from build123d import *

# Parameters (mm, degrees)
SKETCH1_W           = 254
SKETCH1_H           = 38.1
BOSS_EXTRUDE1_DEPTH = 3.175
CUT_EXTRUDE1_DEPTH  = 10.414


with BuildPart() as part:
    # Sketch1 → Boss-Extrude1 (new body)
    with BuildSketch(Plane.XY):
        Rectangle(SKETCH1_W, SKETCH1_H)
    extrude(amount=BOSS_EXTRUDE1_DEPTH)

    # Sketch4 → Cut-Extrude1 (cut)
    with BuildSketch(Plane.XY.offset(3.175)):
        Polygon((-99.060120052, -9.6425385), (-99.060120052, 2.8223845), (-109.855060026, 9.054846), (-120.65, 2.8223845), (-120.65, -9.6425385), (-109.855060026, -15.875), align=None)
        Polygon((-76.200120052, -9.6425385), (-76.200120052, 2.8223845), (-86.995060026, 9.054846), (-97.79, 2.8223845), (-97.79, -9.6425385), (-86.995060026, -15.875), align=None)
        Polygon((-53.340120052, -9.6425385), (-53.340120052, 2.8223845), (-64.135060026, 9.054846), (-74.93, 2.8223845), (-74.93, -9.6425385), (-64.135060026, -15.875), align=None)
        Polygon((-30.480120052, -9.6425385), (-30.480120052, 2.8223845), (-41.275060026, 9.054846), (-52.07, 2.8223845), (-52.07, -9.6425385), (-41.275060026, -15.875), align=None)
        Polygon((120.65, -9.6425385), (120.65, 2.8223845), (109.855060026, 9.054846), (99.060120052, 2.8223845), (99.060120052, -9.6425385), (109.855060026, -15.875), align=None)
        Polygon((97.79, -9.6425385), (97.79, 2.8223845), (86.995060026, 9.054846), (76.200120052, 2.8223845), (76.200120052, -9.6425385), (86.995060026, -15.875), align=None)
    extrude(amount=-CUT_EXTRUDE1_DEPTH, mode=Mode.SUBTRACT)


solid = part.part
Can you work these out from the model? Positions are in its coordinate system, mm. A direction names the side the tool comes from. Round coordinates to 2 decimals unless told otherwise and drop trailing zeros. Loops run counter-clockwise (first coordinate to the right, second up) from the corner with the lowest first, then second, coordinate; pieces in that order, holes last. Notation, with made-up numbers: (3, 65) - (50, 65) arc R4 cw to (50, 70) - close; hole circle Ø10 at (17, 27.25). An arc over 180 degrees is marked (long way). Write item = value, one per line. Start each with the question number.
(1) If we section it at C-C (z = 1.2): Give the number of separate pieces and of enclosed holes in the cut face, and give its area (3 significant figures).
(2) If we section it at B-B (x = -81.5): Please give me the cut outline in (y, z) (3 decimals), and give its area (3 significant figures).
(3) For faces 1 (the face through (-46.748, -12.715, 1.61)), 2 (the face through (-2, 0, 3.175)), which set-ups out of +Z, -Z, +X, -X, +Y, -Y let a thin tool reach every point of the face, with its end or its side?
(4) If I drill on probe 1 along Y at (x, z) = (-57.5, 1.1); probe 2 along Y at (x, z) = (-34.5, 2.65), over which ranges is the centre line in solid material (lowest first)? Write a range as [from, to].
(5) If we section it at D-D (x = 82): Please give me the cut outline in (y, z) (3 decimals), and give its area (3 significant figures).
(6) If we section it at A-A (y = -6.5): Please give me the cut outline in (x, z) (3 decimals), and give its area (3 significant figures).
(7) If we mould it in two halves opening along Y, with no side actions, what happens to faces 3 (the face through (92.32, -12.8, 1.61)), 4 (the face through (-2, 0, 0))? For each: released by +Y, released by -Y, zero draft, split by the parting line, or undercut.
Ans:
q1.separate_pieces = 1
q1.enclosed_holes = 6
q1.area = 7,260 mm²
q2.outline = (-19.05, 0) - (-12.702, 0) - (-12.702, 3.175) - (-19.05, 3.175) - close; (5.882, 0) - (19.05, 0) - (19.05, 3.175) - (5.882, 3.175) - close
q2.area = 62.0 mm²
q3.face_1 = +Z, -Z
q3.face_2 = +Z, +X, -X, +Y, -Y
q4.probe_1 = [-19.05, -12.04], [5.22, 19.05]
q4.probe_2 = [-19.05, -11.96], [5.14, 19.05]
q5.outline = (-19.05, 0) - (-12.991, 0) - (-12.991, 3.175) - (-19.05, 3.175) - close; (6.171, 0) - (19.05, 0) - (19.05, 3.175) - (6.171, 3.175) - close
q5.area = 60.1 mm²
q6.outline = (-127, 0) - (-120.65, 0) - (-120.65, 3.175) - (-127, 3.175) - close; (-99.06, 0) - (-97.79, 0) - (-97.79, 3.175) - (-99.06, 3.175) - close; (-76.2, 0) - (-74.93, 0) - (-74.93, 3.175) - (-76.2, 3.175) - close; (-53.34, 0) - (-52.07, 0) - (-52.07, 3.175) - (-53.34, 3.175) - close; (-30.48, 0) - (76.2, 0) - (76.2, 3.175) - (-30.48, 3.175) - close; (97.79, 0) - (99.06, 0) - (99.06, 3.175) - (97.79, 3.175) - close; (120.65, 0) - (127, 0) - (127, 3.175) - (120.65, 3.175) - close
q6.area = 395 mm²
q7.face_3 = undercut
q7.face_4 = zero draft
